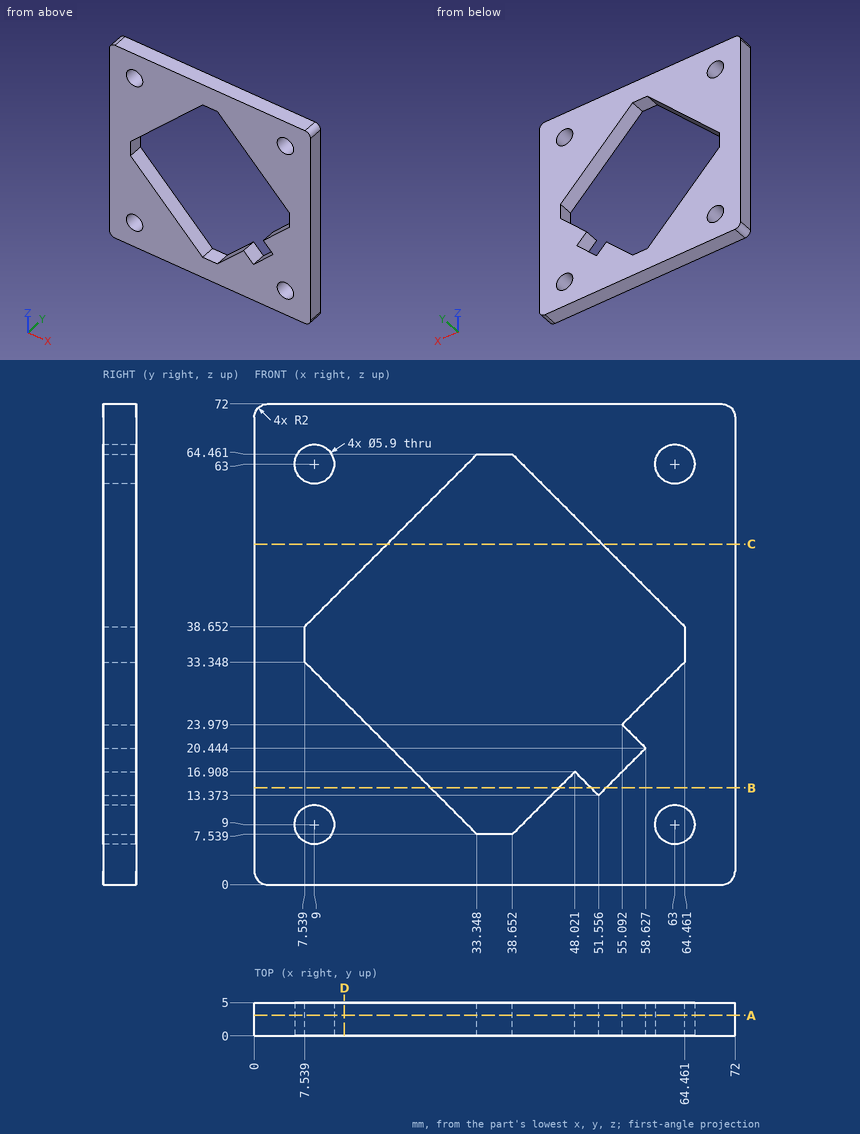
Check sheet for the drawn part. Datum: minimum x, y, z corner. Units: mm. Round coordinates to 2 decimals unless told otherwise and drop trailing zeros. Loops run counter-clockwise (first coordinate to the right, second up) from the corner with the lowest first, then second, coordinate; pieces in that order, holes last.
Item 1: Gauge pin test, flat end, axial feed: pin 1 (1.5 mm diameter, centred on y = 2, z = 18.5, fed in from -X). Record the tip position at first contact, or that the pin passes through.
Item 2: Cross-section at A-A on y = 3.1. Record the boundary of the cut face in (x, z).
Item 3: Cross-section at B-B on z = 14.5. Record the boundary of the cut face in (x, y).
Item 4: Cross-section at D-D on x = 13.5. Record the boundary of the cut face in (y, z), then the cut area to 3 significant figures.
Item 5: Thickness scan on line 1 (Z direction, x = 65.5, y = 1.65) (1 decimal); line 2 (Z direction, x = 57.5, y = 4.5) (1 decimal); line 3 (X direction, y = 0.95, z = 36). Record the ranges inside material, lowest first.
Item 6: Cross-section at C-C on z = 51. Record the boundary of the cut face in (x, y).
Answer sheet:
1. pin 1: stops at x = 0
2. outline: (0, 2) arc R2 ccw to (2, 0) - (70, 0) arc R2 ccw to (72, 2) - (72, 70) arc R2 ccw to (70, 72) - (2, 72) arc R2 ccw to (0, 70) - close; hole circle Ø5.9 at (9, 9); hole circle Ø5.9 at (9, 63); hole (7.54, 33.35) - (33.35, 7.54) - (38.65, 7.54) - (48.02, 16.91) - (51.56, 13.37) - (58.63, 20.44) - (55.09, 23.98) - (64.46, 33.35) - (64.46, 38.65) - (38.65, 64.46) - (33.35, 64.46) - (7.54, 38.65) - close; hole circle Ø5.9 at (63, 9); hole circle Ø5.9 at (63, 63)
3. outline: (0, 0) - (26.39, 0) - (26.39, 5) - (0, 5) - close; (45.61, 0) - (50.43, 0) - (50.43, 5) - (45.61, 5) - close; (52.68, 0) - (72, 0) - (72, 5) - (52.68, 5) - close
4. outline: (0, 0) - (5, 0) - (5, 27.39) - (0, 27.39) - close; (0, 44.61) - (5, 44.61) - (5, 72) - (0, 72) - close
4. area: 274 mm2
5. line 1: z = 0 to 7.4, 10.6 to 61.4, 64.6 to 72
5. line 2: z = 0 to 19.3, 21.6 to 26.4, 45.6 to 72
5. line 3: x = 0 to 7.54, 64.46 to 72
6. outline: (0, 0) - (19.89, 0) - (19.89, 5) - (0, 5) - close; (52.11, 0) - (72, 0) - (72, 5) - (52.11, 5) - close
